```python
from build123d import *

# Parameters (mm, degrees)
SKETCH_W        = 75
SKETCH_H        = 20
PAD_DEPTH       = 15
SKETCH001_W     = 83.048119
SKETCH001_H     = 28.364262
POCKET_DEPTH    = 15.001
SKETCH002_W     = 73.99276
SKETCH002_H     = 21.880196
POCKET001_DEPTH = 13
SKETCH003_R     = 2
POCKET002_DEPTH = 5


with BuildPart() as part:
    # Sketch → Pad (new body)
    with BuildSketch(Plane.XY):
        with Locations((-37.5, -10)):
            Rectangle(SKETCH_W, SKETCH_H)
    extrude(amount=PAD_DEPTH)

    # Sketch001 (on Face6 of Pad) → Pocket (cut, through all)
    with BuildSketch(Plane.XY.offset(15)):
        with Locations((-47.524059, -20.182131)):
            Rectangle(SKETCH001_W, SKETCH001_H)
    extrude(amount=-POCKET_DEPTH, mode=Mode.SUBTRACT)

    # Sketch002 (on Face5 of Pocket) → Pocket001 (cut)
    with BuildSketch(Plane.XY.offset(15)):
        with Locations((-38.99638, -12.940098)):
            Rectangle(SKETCH002_W, SKETCH002_H)
    extrude(amount=-POCKET001_DEPTH, mode=Mode.SUBTRACT)

    # Sketch003 (on Face9 of Pocket001) → Pocket002 (cut)
    with BuildSketch(Plane.XZ.offset(2)):
        with Locations((-13, 7)):
            Circle(SKETCH003_R)
        with Locations((-63, 7)):
            Circle(SKETCH003_R)
        with Locations((-53, 7)):
            Circle(SKETCH003_R)
    extrude(amount=-POCKET002_DEPTH, mode=Mode.SUBTRACT)


solid = part.part
```
Design review of the part built by this model. Coordinates are the model's own, in mm. A direction names the side the tool comes from. Coordinates: 2 decimals unless noted, no trailing zeros. Order: outer loops, then holes, each group sorted by start corner. A loop starts at its lowest first (then second) coordinate and runs counter-clockwise, first axis right, second up. Notation, with made-up numbers: (-31.75, 2.25) -> (-27.75, 2.25) arc R10 cw to (-27.75, 6.25) -> close; hole circle Ø4 at (-3.75, -38.5). An arc over 180 degrees is marked (long way). One line per item, written item: value. Start each with the question number.
Q1. Take a section at C-C, the plane y = -7.75. State the section outline as (x, z) points.
Q2. Insertion check: pin 1 Ø2 at (x, z) = (-46.5, 1.5) entering from -Y; pin 2 Ø2 at (y, z) = (-14.5, 1.5) entering from -X; pin 3 Ø3.5 at (x, z) = (-13, 7) entering from -Y; pin 4 Ø1 at (y, z) = (-8, 7) entering from -X. Each pin has a flat end and moves straight along its axis. Give the tip position at first contact, or say it passes through.
Q3. Tool access review of faces 4 (the flat face through (-38, 0, 7)), 5 (the flat face through (-2, -11, 9)), 6 (the flat face through (-6, -13, 1)): name each direction out of +Z, -Z, +X, -X, +Y, -Y from which nothing blocks a thin tool from reaching the whole face with its end or side.
Q4. Take a section at B-B, the plane z = 7. State the section outline as (x, y) points, then the cut area to 3 significant figures.
Q5. Take a section at D-D, the plane z = 4. State the section outline as (x, y) points, then the cut area to 3 significant figures.
Q6. For probe 1 along Z at (x, y) = (-63, -0.5); probe 2 along Y at (x, z) = (-24, 5), list the stretches that pass through material, from the lowest coordinate up.
Q7. Mouldability with a two-part tool opening along X and no side actions: class faces 1 (the flat face through (-75, -1.7, 5.7)), 2 (the cylindrical face through (-64.474, -1.014, 8.352)), 3 (the flat face through (0, -10, 7)) as pulls with the +X half, pulls with the -X half, needs draft (parallel to the pull), parting line crosses it, or undercut.
Q8. Take a section at A-A, the plane x = -53. State the section outline as (y, z) points, then the cut area to 3 significant figures.
Values follow:
1. outline: (-6, 0) -> (0, 0) -> (0, 15) -> (-2, 15) -> (-2, 2) -> (-6, 2) -> close
2. pin 1: stops at y = -6
2. pin 2: stops at x = -6
2. pin 3: passes through
2. pin 4: stops at x = -2
3. face 4: +Z, -Z, +X, -X, +Y
3. face 5: +Z, -X, -Y
3. face 6: +Z, -Z, -X, -Y
4. outline: (-75, -2) -> (-65, -2) -> (-65, 0) -> (-75, 0) -> close; (-61, -2) -> (-55, -2) -> (-55, 0) -> (-61, 0) -> close; (-51, -2) -> (-15, -2) -> (-15, 0) -> (-51, 0) -> close; (-11, -2) -> (-2, -2) -> (-2, -20) -> (0, -20) -> (0, 0) -> (-11, 0) -> close
4. area: 162 mm2
5. outline: (-75, -2) -> (-2, -2) -> (-2, -20) -> (0, -20) -> (0, 0) -> (-75, 0) -> close
5. area: 186 mm2
6. probe 1: z = 0 to 5, 9 to 15
6. probe 2: y = -2 to 0
7. face 1: pulls with the -X half
7. face 2: undercut
7. face 3: pulls with the +X half
8. outline: (-6, 0) -> (0, 0) -> (0, 5) -> (-2, 5) -> (-2, 2) -> (-6, 2) -> close; (-2, 9) -> (0, 9) -> (0, 15) -> (-2, 15) -> close
8. area: 30.0 mm2
